Design review of the part built by this model. Coordinates are the model's own, in mm. A direction names the side the tool comes from. Round coordinates to 2 decimals unless told otherwise and drop trailing zeros. Loops run counter-clockwise (first coordinate to the right, second up) from the corner with the lowest first, then second, coordinate; pieces in that order, holes last. Notation, with made-up numbers: M 35,26 L 83,26 A25 cw 83,51 Z; hole C -16,-40 d3. An arc over 180 degrees is marked long. Answer as CSV lines item,"result". Start each with the question number.
from build123d import *

# Parameters (mm, degrees)
SKETCH_1_W           = 240
SKETCH_1_H           = 85
EXTRUDE_1_DEPTH      = 25
SKETCH_2_R           = 12
EXTRUDE_2_DEPTH      = 25
SKETCH_3_W           = 233.337502947
SKETCH_3_H           = 53.700186647
CUT_EXTRUDE_1_DEPTH  = 15
SKETCH_4_R           = 12
EXTRUDE_3_DEPTH      = 25
SKETCH_5_W           = 240.131792842
SKETCH_5_H           = 54.002866145
CUT_EXTRUDE_2_DEPTH  = 15
EXTRUDE_4_DEPTH      = 5
EXTRUDE_4_DEPTH_BACK = 25
SKETCH_6_R           = 12
SKETCH_8_R           = 28
EXTRUDE_5_DEPTH      = 60
SKETCH_9_W           = 240
SKETCH_9_H           = 25
EXTRUDE_6_DEPTH      = 70
SKETCH_10_W          = 36
SKETCH_10_H          = 40
EXTRUDE_7_DEPTH      = 15
SKETCH_11_R          = 10
CUT_EXTRUDE_3_DEPTH  = 10


with BuildPart() as part:
    # 草图1 → 凸台-拉伸1 (new body)
    with BuildSketch(Plane.XY):
        with Locations((120, 42.5)):
            Rectangle(SKETCH_1_W, SKETCH_1_H)
    extrude(amount=EXTRUDE_1_DEPTH)

    # 草图2 → 凸台-拉伸2 (add)
    # profile 1 of 2: a face of its own
    with BuildSketch(Plane.XZ):
        with BuildLine():
            Line((0, 0), (30, 0))
            Line((30, 0), (60, 0))
            Line((60, 0), (49.138858248, -35.805524564))
            ThreePointArc((49.138858248, -35.805524564), (30, -50.000000263), (10.861141752, -35.805524564))
            Line((10.861141752, -35.805524564), (0, 0))
        make_face()
        with Locations(Location((30, -30, 0), (0, 0, 270))):
            Circle(SKETCH_2_R, mode=Mode.SUBTRACT)
    # profile 2 of 2: a face of its own
    with BuildSketch(Plane.XZ):
        with BuildLine():
            Line((170, 0), (230, 0))
            Line((230, 0), (219.138858248, -35.805524564))
            ThreePointArc((219.138858248, -35.805524564), (200, -50.000000263), (180.861141752, -35.805524564))
            Line((180.861141752, -35.805524564), (170, 0))
        make_face()
        with Locations(Location((200, -30, 0), (0, 0, 270))):
            Circle(SKETCH_2_R, mode=Mode.SUBTRACT)
    extrude(amount=-EXTRUDE_2_DEPTH)

    # 草图3 → 切除-拉伸1 (cut)
    with BuildSketch(Plane(origin=(0, 5, 0), x_dir=(-1, 0, 0), z_dir=(0, -1, 0))):
        with Locations((-113.331248527, 26.850093324)):
            Rectangle(SKETCH_3_W, SKETCH_3_H)
    extrude(amount=-CUT_EXTRUDE_1_DEPTH, mode=Mode.SUBTRACT)

    # 草图4 → 凸台-拉伸3 (add)
    # profile 1 of 2: a face of its own
    with BuildSketch(Plane(origin=(0, 85, 0), x_dir=(1, 0, 0), z_dir=(0, 1, 0))):
        with BuildLine():
            Line((20.861141752, 35.805524564), (10, 0))
            Line((10, 0), (70, 0))
            Line((70, 0), (59.138858248, 35.805524564))
            ThreePointArc((59.138858248, 35.805524564), (40, 50.000000263), (20.861141752, 35.805524564))
        make_face()
        with Locations(Location((40, 30, 0), (0, 0, 270))):
            Circle(SKETCH_4_R, mode=Mode.SUBTRACT)
    # profile 2 of 2: a face of its own
    with BuildSketch(Plane(origin=(0, 85, 0), x_dir=(1, 0, 0), z_dir=(0, 1, 0))):
        with BuildLine():
            Line((190.861141752, 35.805524564), (180, 0))
            Line((180, 0), (240, 0))
            Line((240, 0), (229.138858248, 35.805524564))
            ThreePointArc((229.138858248, 35.805524564), (210, 50.000000263), (190.861141752, 35.805524564))
        make_face()
        with Locations(Location((210, 30, 0), (0, 0, 270))):
            Circle(SKETCH_4_R, mode=Mode.SUBTRACT)
    extrude(amount=-EXTRUDE_3_DEPTH)

    # 草图5 → 切除-拉伸2 (cut)
    with BuildSketch(Plane(origin=(0, 80, 0), x_dir=(1, 0, 0), z_dir=(0, 1, 0))):
        with Locations((130.065896421, 27.001433073)):
            Rectangle(SKETCH_5_W, SKETCH_5_H)
    extrude(amount=-CUT_EXTRUDE_2_DEPTH, mode=Mode.SUBTRACT)

    # 草图6 → 凸台-拉伸4 (add, two sides: drawn at the far end of the back side and taken through both)
    with BuildSketch(Plane.XZ.offset(-EXTRUDE_4_DEPTH_BACK)):
        with Locations(Location((200, -30, 0), (0, 0, 90))):
            Circle(SKETCH_6_R)
    extrude(amount=EXTRUDE_4_DEPTH + EXTRUDE_4_DEPTH_BACK)

    # 草图8 → 凸台-拉伸5 (add)
    with BuildSketch(Plane.XZ.offset(5)):
        with Locations(Location((200, -30, 0), (0, 0, 270))):
            Circle(SKETCH_8_R)
    extrude(amount=EXTRUDE_5_DEPTH)

    # 草图9 → 凸台-拉伸6 (add)
    with BuildSketch(Plane.XZ):
        with Locations((120, 12.5)):
            Rectangle(SKETCH_9_W, SKETCH_9_H)
    extrude(amount=EXTRUDE_6_DEPTH)

    # 草图10 → 凸台-拉伸7 (add)
    with BuildSketch(Plane(origin=(0, 0, 0), x_dir=(-1, 0, 0), z_dir=(0, 0, -1))):
        with Locations((-200, -35)):
            Rectangle(SKETCH_10_W, SKETCH_10_H)
    extrude(amount=EXTRUDE_7_DEPTH)

    # 草图11 → 切除-拉伸3 (cut)
    with BuildSketch(Plane.XZ.offset(70)):
        with Locations(Location((50, 12.5, 0), (0, 0, 270))):
            Circle(SKETCH_11_R)
        with Locations(Location((190, 12.5, 0), (0, 0, 270))):
            Circle(SKETCH_11_R)
    extrude(amount=-CUT_EXTRUDE_3_DEPTH, mode=Mode.SUBTRACT)


solid = part.part
Item 1: Tool access review of faces 1 (the face through (200, 22, -50)), 2 (the face through (200, 20, -14)), 3 (the face through (210, 63, -50)), 4 (the face through (30, 2, -50)): name each direction out of +Z, -Z, +X, -X, +Y, -Y from which nothing blocks a thin tool from reaching the whole face with its end or side.
Item 2: Consider section D-D, the plane x = 67. Write out the cut boundary in (y, z).
Item 3: Consider section B-B, the plane x = 207.5. Count the separate pieces of the cut face and the enclosed holes in it, then the cut area to 3 significant figures.
Item 4: Consider section A-A, the plane y = -35.5. Write out the cut boundary in (x, z).
Item 5: Insertion check: pin 1 Ø25 at (x, z) = (44, -23) entering from -Y; pin 2 Ø1 at (x, z) = (198.5, -38) entering from -Y; pin 3 Ø3 at (y, z) = (-48, -22.5) entering from +X. Each pin has a flat end and moves straight along its axis. Give the tip position at first contact, or say it passes through.
Item 6: To check wall thickness, follow line 1 (X direction, y = -65, z = 12); line 2 (Y direction, x = 176.5, z = -8); line 3 (Y direction, x = 57.5, z = -34). State the ranges of each line that lie inside material, in increasing order.
Item 7: The part is to be moulded in two halves that separate along Y. For faces 5 (the face through (200, 25, -19)), 6 (the face through (200, -55, -1)), 7 (the face through (175.507, 22.465, -18.153)), say which applies: +Y half, -Y half, draft (parallel to the pull), parting line (faces both ways), or undercut.
Found:
1,face 1,"-Z"
1,face 2,"none"
1,face 3,"-Z, +Y"
1,face 4,"-Z, -Y"
2,outline,"M -70,0 L 60,0 L 60,-9.89 L 65,-9.89 L 65,0 L 80,0 L 80,-9.89 L 85,-9.89 L 85,25 L -70,25 Z"
3,separate pieces,"3"
3,enclosed holes,"2"
3,area,"8,360 mm^2"
4,outline,"M 0,0 L 182,0 L 182,-8.55 A28 ccw long 218,-8.55 L 218,0 L 240,0 L 240,25 L 0,25 Z"
5,pin 1,"stops at y = 0"
5,pin 2,"stops at y = -65"
5,pin 3,"stops at x = 227.35"
6,line 1,"x = 0 to 40.01, 59.99 to 180.01, 199.99 to 240"
6,line 2,"y = 0 to 5, 20 to 25"
6,line 3,"y = 60 to 65, 80 to 85"
7,face 5,"undercut"
7,face 6,"-Y half"
7,face 7,"draft"
